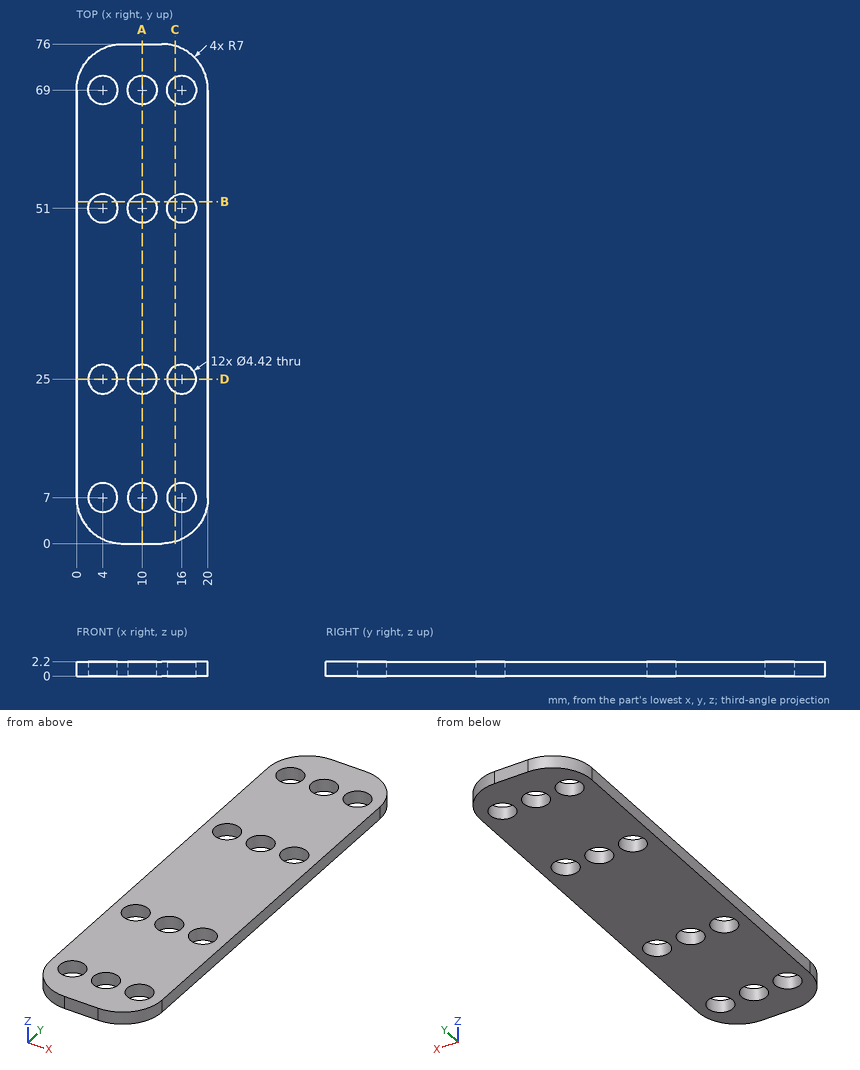
For this review, use the dimensioned drawing (mm, ordinates from the lowest corner) and the shaded views. Coordinates: 2 decimals unless noted, no trailing zeros. Order: outer loops, then holes, each group sorted by start corner. A loop starts at its lowest first (then second) coordinate and runs counter-clockwise, first axis right, second up. Notation, with made-up numbers: (-36.5, 72) - (-0.5, 72) arc R20 cw to (-0.5, 93) - close; hole circle Ø9 at (22.5, 20.25). An arc over 180 degrees is marked (long way). Answer as a JSON object with one key per item and string values. Group by question number.
1. We need section A-A on x = 10. State the section outline as (y, z) points, then the cut area to 3 significant figures.
2. We need section B-B on y = 52. State the section outline as (x, z) points.
3. We need section D-D on y = 25. State the section outline as (x, z) points.
4. We need section C-C on x = 15. State the section outline as (y, z) points, then the cut area to 3 significant figures.
5. Clearance check with a flat-ended pin moving along its axis: P1, Ø3.5, axis at x = 16, y = 51, coming from the +Z side. State where the tip first meets the part, or that it passes through.
6. For probe 1 along X at (y, z) = (69, 1.05); probe 2 along Y at (x, z) = (4, 1.6); probe 3 along Y at (x, z) = (3, 1.2), list the stretches that pass through material, from the lowest coordinate up.
Final values:
{
 "1": {"outline": "(0, 0) - (4.79, 0) - (4.79, 2.2) - (0, 2.2) - close; (9.21, 0) - (22.79, 0) - (22.79, 2.2) - (9.21, 2.2) - close; (27.21, 0) - (48.79, 0) - (48.79, 2.2) - (27.21, 2.2) - close; (53.21, 0) - (66.79, 0) - (66.79, 2.2) - (53.21, 2.2) - close; (71.21, 0) - (76, 0) - (76, 2.2) - (71.21, 2.2) - close", "area": "128 mm²"},
 "2": {"outline": "(0, 0) - (2.03, 0) - (2.03, 2.2) - (0, 2.2) - close; (5.97, 0) - (8.03, 0) - (8.03, 2.2) - (5.97, 2.2) - close; (11.97, 0) - (14.03, 0) - (14.03, 2.2) - (11.97, 2.2) - close; (17.97, 0) - (20, 0) - (20, 2.2) - (17.97, 2.2) - close"},
 "3": {"outline": "(0, 0) - (1.79, 0) - (1.79, 2.2) - (0, 2.2) - close; (6.21, 0) - (7.79, 0) - (7.79, 2.2) - (6.21, 2.2) - close; (12.21, 0) - (13.79, 0) - (13.79, 2.2) - (12.21, 2.2) - close; (18.21, 0) - (20, 0) - (20, 2.2) - (18.21, 2.2) - close"},
 "4": {"outline": "(0.29, 0) - (5.03, 0) - (5.03, 2.2) - (0.29, 2.2) - close; (8.97, 0) - (23.03, 0) - (23.03, 2.2) - (8.97, 2.2) - close; (26.97, 0) - (49.03, 0) - (49.03, 2.2) - (26.97, 2.2) - close; (52.97, 0) - (67.03, 0) - (67.03, 2.2) - (52.97, 2.2) - close; (70.97, 0) - (75.71, 0) - (75.71, 2.2) - (70.97, 2.2) - close", "area": "131 mm²"},
 "5": {"P1": "through"},
 "6": {"probe 1": "0 to 1.79, 6.21 to 7.79, 12.21 to 13.79, 18.21 to 20", "probe 2": "0.68 to 4.79, 9.21 to 22.79, 27.21 to 48.79, 53.21 to 66.79, 71.21 to 75.32", "probe 3": "1.26 to 5.03, 8.97 to 23.03, 26.97 to 49.03, 52.97 to 67.03, 70.97 to 74.74"}
}
